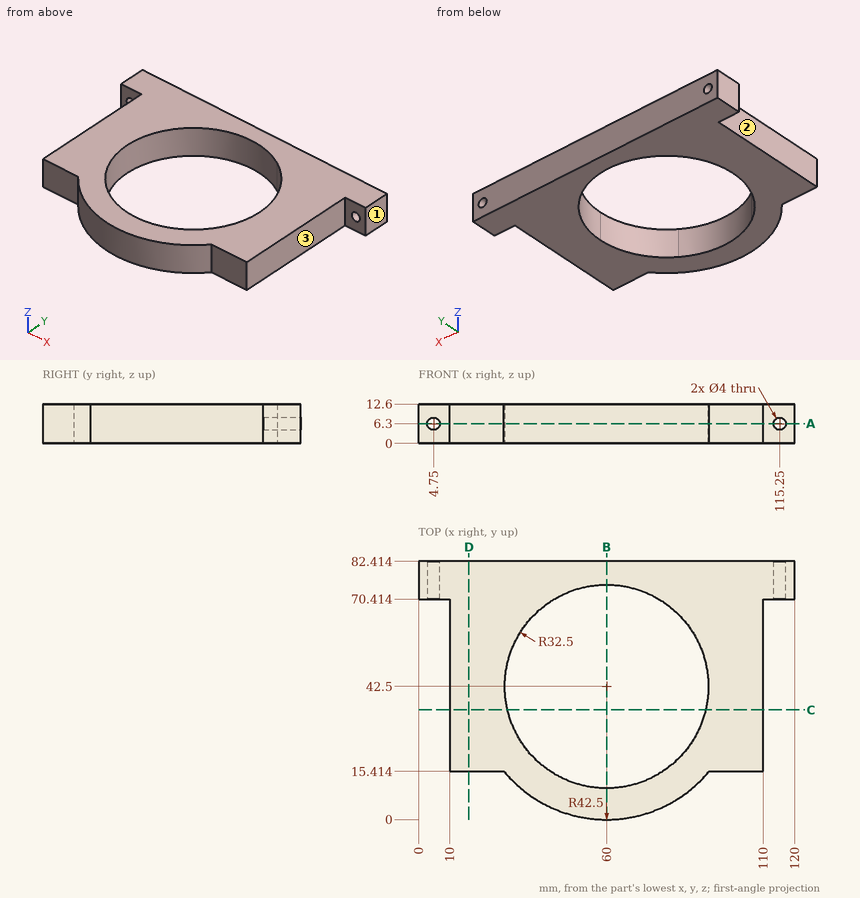
Here's the drawing with two shaded views (mm, measured from the low corner). I have some questions. A direction names the side the tool comes from. Round coordinates to 2 decimals unless told otherwise and drop trailing zeros. Loops run counter-clockwise (first coordinate to the right, second up) from the corner with the lowest first, then second, coordinate; pieces in that order, holes last. Notation, with made-up numbers: (66.5, 20) - (107.5, 20) arc R22 cw to (107.5, 34) - close; hole circle Ø8 at (-1.75, 17). An arc over 180 degrees is marked (long way). Use CSV: the item, a comma, the result in double quotes. Start each with the question number.
1) If we section it at D-D on x = 16: Write out the boundary of the cut face in (y, z), plus the area to 3 significant figures.
2) For pin 1 Ø6.5 at (x, z) = (97.5, 3.5) entering from -Y; pin 2 Ø5 at (y, z) = (42, 5.5) entering from +X; pin 3 Ø6 at (y, z) = (19, 5.5) entering from -X, each with a flat end and sliding along its axis, tell me the tip position at first contact or that it passes through.
3) For the marked faces 1, 2 and 3, which set-ups out of +Z, -Z, +X, -X, +Y, -Y let a thin tool reach every point of the face, with its end or its side?
4) If we section it at B-B on x = 60: Write out the boundary of the cut face in (y, z), plus the area to 3 significant figures.
5) If we section it at C-C on y = 35: Write out the boundary of the cut face in (x, z), plus the area to 3 significant figures.
6) Please list where these lines run through material, in increasing order: probe 1 along Z at (x, y) = (115.25, 73); probe 2 along Y at (x, z) = (74, 6.5); probe 3 along Y at (x, z) = (12.5, 1.25). Write a range as [from, to].
7) If we section it at A-A on z = 6.3: Write out the boundary of the cut face in (x, y).
Geometry results:
1,outline,"(15.41, 0) - (82.41, 0) - (82.41, 12.6) - (15.41, 12.6) - close"
1,area,"844 mm2"
2,pin 1,"stops at y = 15.41"
2,pin 2,"stops at x = 110"
2,pin 3,"stops at x = 10"
3,face 1,"+Z, -Z, +X, +Y, -Y"
3,face 2,"+Z, -Z, -X, -Y"
3,face 3,"+Z, -Z, +X, -Y"
4,outline,"(0, 0) - (10, 0) - (10, 12.6) - (0, 12.6) - close; (75, 0) - (82.41, 0) - (82.41, 12.6) - (75, 12.6) - close"
4,area,"219 mm2"
5,outline,"(10, 0) - (28.38, 0) - (28.38, 12.6) - (10, 12.6) - close; (91.62, 0) - (110, 0) - (110, 12.6) - (91.62, 12.6) - close"
5,area,"463 mm2"
6,probe 1,"z = [0, 4.3], [8.3, 12.6]"
6,probe 2,"y = [2.37, 13.17], [71.83, 82.41]"
6,probe 3,"y = [15.41, 82.41]"
7,outline,"(0, 70.41) - (2.75, 70.41) - (2.75, 82.41) - (0, 82.41) - close; (6.75, 70.41) - (10, 70.41) - (10, 15.41) - (27.25, 15.41) arc R42.5 ccw to (92.75, 15.41) - (110, 15.41) - (110, 70.41) - (113.25, 70.41) - (113.25, 82.41) - (6.75, 82.41) - close; (117.25, 70.41) - (120, 70.41) - (120, 82.41) - (117.25, 82.41) - close; hole circle Ø65 at (60, 42.5)"
